Autodesk Inventor part; units mm, degrees
ref_plane "YZ Plane" through (0, 0, 0) normal (1, 0, 0) x (0, 1, 0)
ref_plane "XZ Plane" through (0, 0, 0) normal (0, 1, 0) x (-1, 0, 0)
ref_plane "XY Plane" through (0, 0, 0) normal (0, 0, 1) x (1, 0, 0)
sketch "Sketch1" plane through (0, 0, 0) normal (0, 1, 0) x (-1, 0, 0)
  line L0 (-2, -2) -> (-22, -2) construction
  line L1 (-2, 3) -> (-22, 3)
  line L2 (-22, -7) -> (-2, -7)
  arc A0 (-2, -7) -> (-2, 3) centre (-2, -2) ccw
  arc A1 (-22, 3) -> (-22, -7) centre (-22, -2) ccw
  circle A2 centre (-2, -2) radius 2.5
  circle A3 centre (-22, -2) radius 2.5
  point P0 (0, 0)
  point P1 (-12, -2)
  dimension "d0" = 20
  dimension "d1" = 10
  dimension "d2" = 5
extrude "Extrusion1" add sketch "Sketch1" along normal blind 5 contours A0 L2 A1 L1 | A2
sketch "Sketch2" plane through (0, 5, 0) normal (0, 1, 0) x (1, 0, 0)
  circle A0 centre (2, 2) radius 2.5
  point P0 (0, 0)
extrude "Extrusion3" add sketch "Sketch2" along normal blind 5
Work out the finished part from the listing and answer in its coordinate system (mm). A direction names the side the tool comes from. Coordinates: 2 decimals unless noted, no trailing zeros. Order: outer loops, then holes, each group sorted by start corner. A loop starts at its lowest first (then second) coordinate and runs counter-clockwise, first axis right, second up. Notation, with made-up numbers: (12, 74.25) - (64, 74.25) arc R17 ccw to (64, 87.25) - close; hole circle Ø5 at (16, 4). An arc over 180 degrees is marked (long way). Put each result on its own line as item: value. Start each with the question number.
1) Find the intervals of material crossed by line 1 (Z direction, x = 22, y = 2.3); line 2 (Y direction, x = 10.5, z = -1.25); line 3 (Z direction, x = 21.5, y = 0.5), in increasing order. Write a range as from..to.
2) Find section A-A (z = -2). Give the vertices of the cut face in (x, y), plus the area to 3 significant figures.
3) Find section C-C (z = 1). Give the vertices of the cut face in (x, y).
4) Find section B-B (y = 3). Give the vertices of the cut face in (x, z), plus the area to 3 significant figures.
5) For a pull along X with two mould halves and no side action, classify faces 3 (the flat face through (12, 2, 3)), 4 (the cylindrical face through (24.5, 2.5, -2.1)), 5 (the cylindrical face through (-3, 2, -2)) as released by +X, released by -X, zero draft, split by the parting line, or undercut.
6) Find section D-D (x = 8). Give the vertices of the cut face in (y, z).
7) For faces 1 (the cylindrical face through (-0.5, 7.5, -1.9)), 2 (the flat face through (2, 10, -2)), determine the directions among +Z, -Z, +X, -X, +Y, -Y from which every point of the face is accessible in a straight line to the end or side of a thin tool.
Results list:
1. line 1: z = -7..-4.5, 0.5..3
1. line 2: y = 0..5
1. line 3: z = -7..-4.45, 0.45..3
2. outline: (-3, 0) - (19.5, 0) - (19.5, 5) - (4.5, 5) - (4.5, 10) - (-0.5, 10) - (-0.5, 5) - (-3, 5) - close; (24.5, 0) - (27, 0) - (27, 5) - (24.5, 5) - close
2. area: 150 mm^2
3. outline: (-2, 0) - (26, 0) - (26, 5) - (-2, 5) - close
4. outline: (2, -7) - (22, -7) arc R5 ccw to (22, 3) - (2, 3) arc R5 ccw to start; hole circle Ø5 at (22, -2)
4. area: 259 mm^2
5. face 3: zero draft
5. face 4: undercut
5. face 5: released by -X
6. outline: (0, -7) - (5, -7) - (5, 3) - (0, 3) - close
7. face 1: +Y
7. face 2: +Z, -Z, +X, -X, +Y
